Here's how the part is built. I have some questions about the finished solid (model axes, mm). Face numbers are marked on the shaded views. Coordinates: 2 decimals unless noted, no trailing zeros. Order: outer loops, then holes, each group sorted by start corner. A loop starts at its lowest first (then second) coordinate and runs counter-clockwise, first axis right, second up.
```python
from build123d import *

# Parameters (mm, degrees)
F0_W     = 103
F0_H     = 103
F1_DEPTH = 100
F2_W     = 97
F2_H     = 97
F3_DEPTH = 97
F4_W     = 1
F4_H     = 19
F4_W_2   = 19
F4_H_2   = 1
F5_DEPTH = 5


with BuildPart() as f1:
    # F0 (on Top) → F1 (new body)
    with BuildSketch(Plane.XY):
        with Locations((51.5, 51.5)):
            Rectangle(F0_W, F0_H)
    extrude(amount=F1_DEPTH)

    # F2 (on face) → F3 (cut)
    with BuildSketch(Plane.XY.offset(100)):
        with Locations((51.5, 51.5)):
            Rectangle(F2_W, F2_H)
    extrude(amount=-F3_DEPTH, mode=Mode.SUBTRACT)

    # F4 (on face) → F5 (cut)
    with BuildSketch(Plane.XY.offset(100)):
        Polygon((21, 102), (1, 102), (1, 101), (2, 101), (21, 101), align=None)
        with Locations((1.5, 91.5)):
            Rectangle(F4_W, F4_H)
        Polygon((2, 21), (1, 21), (1, 1), (2, 1), (2, 2), align=None)
        with Locations((11.5, 1.5)):
            Rectangle(F4_W_2, F4_H_2)
        Polygon((101, 2), (82, 2), (82, 1), (102, 1), (102, 2), align=None)
        with Locations((101.5, 11.5)):
            Rectangle(F4_W, F4_H)
        Polygon((102, 102), (82, 102), (82, 101), (101, 101), (102, 101), align=None)
        with Locations((101.5, 91.5)):
            Rectangle(F4_W, F4_H)
    extrude(amount=-F5_DEPTH, mode=Mode.SUBTRACT)


solid = f1.part
```
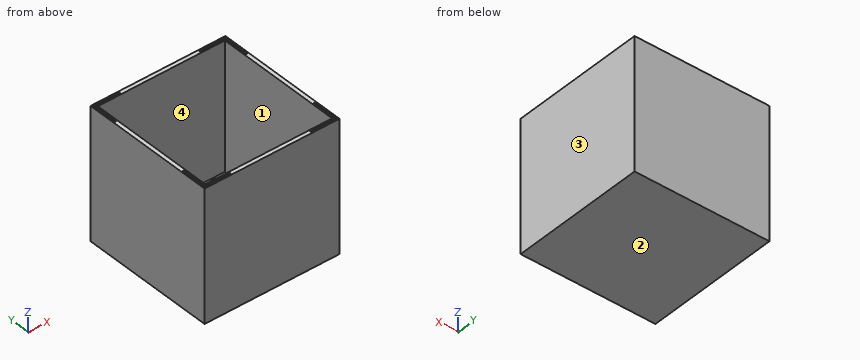
Q1. We'd pull the mould along X, two halves only. Please class the marked faces 1, 2, 3 and 4: pulls with the +X half, pulls with the -X half, needs draft (parallel to the pull), parting line crosses it, or undercut.
Q2. Will this pin go through, and if not, where does the flat tip stop? pin 1 (3 mm diameter, centred on x = 40, y = 81, fed in from +Z).
Q3. I need wall thicknesses on L1, parallel to Y at x = 75.5, z = 76; L2, parallel to Z at x = 34, y = 56.5. Which ranges of each line are inside material? Lowest first, please.
Q4. If we section it at A-A on z = 32: Write out the boundary of the cut face in (x, y), then the cut area to 3 significant figures.
Q5. If we section it at C-C on y = 32: Write out the boundary of the cut face in (x, z).
Q6. If we section it at B-B on x = 10.5: Write out the boundary of the cut face in (y, z), then the cut area to 3 significant figures.
Reply:
1. face 1: undercut
1. face 2: needs draft
1. face 3: pulls with the +X half
1. face 4: undercut
2. pin 1: stops at z = 3
3. L1: y = 0 to 3, 100 to 103
3. L2: z = 0 to 3
4. outline: (0, 0) - (103, 0) - (103, 103) - (0, 103) - close; hole (3, 3) - (100, 3) - (100, 100) - (3, 100) - close
4. area: 1,200 mm2
5. outline: (0, 0) - (103, 0) - (103, 100) - (100, 100) - (100, 3) - (3, 3) - (3, 100) - (0, 100) - close
6. outline: (0, 0) - (103, 0) - (103, 100) - (102, 100) - (102, 95) - (101, 95) - (101, 100) - (100, 100) - (100, 3) - (3, 3) - (3, 100) - (2, 100) - (2, 95) - (1, 95) - (1, 100) - (0, 100) - close
6. area: 881 mm2
